```python
from build123d import *

# Parameters (mm, degrees)
F0_W     = 106
F0_H     = 87
F1_DEPTH = 12
F2_R     = 3
F3_DEPTH = 20
F5_DEPTH = 20
F6_DEPTH = 20
F7_R     = 2
F8_DEPTH = 10


with BuildPart() as f1:
    # F0 (on Right) → F1 (new body)
    with BuildSketch(Plane.YZ):
        with Locations((53, 43.5)):
            Rectangle(F0_W, F0_H)
    extrude(amount=F1_DEPTH)

    # F2 (on face) → F3 (cut)
    with BuildSketch(Plane.XY.offset(87)):
        with Locations((6, 88)):
            Circle(F2_R)
        with Locations((6, 48)):
            Circle(F2_R)
        with Locations((6, 8)):
            Circle(F2_R)
    extrude(amount=-F3_DEPTH, mode=Mode.SUBTRACT)

    # F2 (on face) → F5 (cut)
    with BuildSketch(Plane.XY.offset(87)):
        with Locations((6, 88)):
            Circle(F2_R)
        with Locations((6, 48)):
            Circle(F2_R)
        with Locations((6, 8)):
            Circle(F2_R)
    extrude(amount=-F5_DEPTH, mode=Mode.SUBTRACT)

    # F4 (on face) → F6 (cut)
    with BuildSketch(Plane(origin=(0, 0, 0), x_dir=(1, 0, 0), z_dir=(0, 0, -1))):
        with BuildLine():
            ThreePointArc((6, -85), (3, -88), (6, -91))
            Line((6, -91), (6, -88))
            Line((6, -88), (6, -85))
        make_face()
        with BuildLine():
            ThreePointArc((6, -5), (3, -8), (6, -11))
            Line((6, -11), (6, -5))
        make_face()
        with BuildLine():
            Line((6, -5), (6, -11))
            ThreePointArc((6, -11), (8.12132, -10.12132), (9, -8))
            ThreePointArc((9, -8), (8.12132, -5.87868), (6, -5))
        make_face()
        with BuildLine():
            ThreePointArc((6, -45), (3, -48), (6, -51))
            Line((6, -51), (6, -48))
            Line((6, -48), (6, -45))
        make_face()
        with BuildLine():
            Line((6, -48), (6, -51))
            ThreePointArc((6, -51), (8.12132, -50.12132), (9, -48))
            ThreePointArc((9, -48), (8.12132, -45.87868), (6, -45))
            Line((6, -45), (6, -48))
        make_face()
        with BuildLine():
            Line((6, -88), (6, -91))
            ThreePointArc((6, -91), (8.12132, -90.12132), (9, -88))
            Line((9, -88), (6, -88))
        make_face()
        with BuildLine():
            Line((6, -85), (6, -88))
            Line((6, -88), (9, -88))
            ThreePointArc((9, -88), (8.12132, -85.87868), (6, -85))
        make_face()
    extrude(amount=-F6_DEPTH, mode=Mode.SUBTRACT)

    # F7 (on face) → F8 (cut)
    with BuildSketch(Plane(origin=(0, 106, 0), x_dir=(-1, 0, 0), z_dir=(0, 1, 0))):
        with Locations((-6, 77)):
            Circle(F7_R)
        with Locations((-6, 10)):
            Circle(F7_R)
    extrude(amount=-F8_DEPTH, mode=Mode.SUBTRACT)


solid = f1.part
```
Design review of the part built by this model. Coordinates are the model's own, in mm. A direction names the side the tool comes from. Give positions to 0.01 mm unless a question says otherwise; leave off trailing zeros. Write each loop counter-clockwise with the first axis right and the second up, starting at its lowest first coordinate (ties: lowest second). Pieces come first, ordered by that corner, then holes. Notation, with made-up numbers: (49, -16.75) - (100, -16.75) arc R9 cw to (100, -7.75) - close; hole circle Ø4 at (48.25, 42.25). An arc over 180 degrees is marked (long way). Return JSON: item names as keys, results as strings. Group by question number.
(1) Mouldability with a two-part tool opening along Y and no side actions: class faces 1 (the flat face through (6, 8, 20)), 2 (the flat face through (6, 106, 43)), 3 (the cylindrical face through (6, 101, 12)) as +Y half, -Y half, draft (parallel to the pull), parting line (faces both ways), or undercut.
(2) We need section A-A, the plane z = 70. Give the boundary of the cut face in (x, y), then the cut area to 3 significant figures.
(3) To check wall thickness, follow probe 1 along Z at (x, y) = (6, 100); probe 2 along Y at (x, z) = (6, 72.25); probe 3 along Y at (x, z) = (8.75, 6.5). State the ranges of each line that lie inside material, in increasing order.
(4) We need section B-B, the plane z = 10. Give the boundary of the cut face in (x, y), then the cut area to 3 significant figures.
(5) Machinability: for faces 4 (the flat face through (6, 8, 67)), 5 (the flat face through (12, 52, 44)), 6 (the flat face through (6, 96, 77)), 7 (the flat face through (6, 52, 87)), 8 (the flat face through (6, 88, 20)), which of the approach directions +Z, -Z, +X, -X, +Y, -Y give a long, thin tool a straight path to every point of the face, cutting with its end or side? Answer none if there is none.
(6) Insertion check: pin 1 (1.8 mm diameter, centred on x = 7.5, y = 7.5, fed in from -Z); pin 2 (3 mm diameter, centred on x = 7, y = 8, fed in from +Z); pin 3 (3 mm diameter, centred on x = 6, z = 77, fed in from +Y). Each pin has a flat end and moves straight along its axis. Give the tip position at first contact, or say it passes through.
Reported:
{
 "1": {"face 1": "undercut", "face 2": "+Y half", "face 3": "draft"},
 "2": {"outline": "(0, 0) - (12, 0) - (12, 106) - (0, 106) - close; hole circle Ø6 at (6, 8); hole circle Ø6 at (6, 48); hole circle Ø6 at (6, 88)", "area": "1,190 mm2"},
 "3": {"probe 1": "z = 0 to 8, 12 to 75, 79 to 87", "probe 2": "y = 0 to 5, 11 to 45, 51 to 85, 91 to 106", "probe 3": "y = 0 to 6.8, 9.2 to 46.8, 49.2 to 86.8, 89.2 to 106"},
 "4": {"outline": "(0, 0) - (12, 0) - (12, 106) - (8, 106) - (8, 96) - (4, 96) - (4, 106) - (0, 106) - close; hole (6, 5) arc R3 ccw to (9, 8) arc R3 ccw to (6, 11) arc R3 ccw to start; hole (6, 45) arc R3 ccw to (9, 48) arc R3 ccw to (6, 51) arc R3 ccw to start; hole (6, 85) arc R3 ccw to (9, 88) arc R3 ccw to (6, 91) arc R3 ccw to start", "area": "1,150 mm2"},
 "5": {"face 4": "+Z", "face 5": "+Z, -Z, +X, +Y, -Y", "face 6": "+Y", "face 7": "+Z, +X, -X, +Y, -Y", "face 8": "-Z"},
 "6": {"pin 1": "stops at z = 20", "pin 2": "stops at z = 67", "pin 3": "stops at y = 96"}
}
